```python
from build123d import *


with BuildPart() as f1:
    # F0 (on Top) → F1 (revolve)
    with BuildSketch(Plane.XY):
        Polygon((0, 76.635234), (0, -54.980509), (15.186432, -54.980509), (15.186432, -38.387928), (55.121128, -38.387928), (33.747628, -14.202126), (57.652198, -14.202126), (33.747628, 13.077206), (55.121128, 13.077206), (33.747628, 36.419317), (51.183905, 36.419317), align=None)
    revolve(axis=Axis((0, 10.827363, 0), (0, -1, 0)))


solid = f1.part
```
Geometry check sheet. Reference: the model listing, model coordinates, mm. A direction names the side the tool comes from. Round coordinates to 2 decimals unless told otherwise and drop trailing zeros. Loops run counter-clockwise (first coordinate to the right, second up) from the corner with the lowest first, then second, coordinate; pieces in that order, holes last. Notation, with made-up numbers: (-34, -26) - (25, -26) arc R32 cw to (25, 7) - close; hole circle Ø11 at (11.25, 77). An arc over 180 degrees is marked (long way). Write item = value, one per line. Start each with the question number.
1. Section check B-B on z = 35. Give the number of separate pieces and of enclosed holes in the cut face, then the cut area to 3 significant figures.
2. Section check C-C on y = -44. Enter the section's corners in (x, z), then the cut area to 3 significant figures.
3. Mould release check, pull along Y, two halves, no side actions. Record for faces 4 (the face through (7.8, 70.2, 2.5)), 5 (the face through (-7.541, 35.286, -33.958)), 6 (the face through (-12.05, -46.57, -9.24)): released by +Y, released by -Y, zero draft, split by the parting line, or undercut.
4. Section check A-A on y = 17.5. Enter the section's corners in (x, z).
5. Depth check by flat-ended pin: pin 1 (1.5 mm diameter, centred on x = 29, z = -44, fed in from -Y); pin 2 (8 mm diameter, centred on y = 57, z = -24.5, fed in from -X); pin 3 (5 mm diameter, centred on x = -7.5, z = -10.5, fed in from +Y). Enter the tip coordinate at first touch or a pass-through.
6. Set-up check for faces 1 (the face through (0, -54.981, 0)), 2 (the face through (-11, 36.419, -33)), 3 (the face through (-11, -38.388, -11)): record each of +Z, -Z, +X, -X, +Y, -Y from which the full face is reachable in a straight line by a thin tool's end or side.
7. Thickness scan on line 1 (Y direction, x = -23.5, z = 27); line 2 (Y direction, x = -34, z = -39); line 3 (Y direction, x = -36.5, z = -22). Record the ranges inside material, lowest first.
Working result:
q1.separate_pieces = 4
q1.enclosed_holes = 0
q1.area = 4,530 mm^2
q2.outline = circle Ø30.37 at (0, 0)
q2.area = 725 mm^2
q3.face_4 = released by +Y
q3.face_5 = undercut
q3.face_6 = zero draft
q4.outline = circle Ø102.14 at (0, 0)
q5.pin_1 = -38.39
q5.pin_2 = -18.92
q5.pin_3 = 68.46
q6.face_1 = +Z, -Z, +X, -X, -Y
q6.face_2 = none
q6.face_3 = -Y
q7.line_1 = -38.39 to -16.52, -14.2 to 10.74, 13.08 to 34.18, 36.42 to 48.51
q7.line_2 = -38.39 to -34.56, -14.2 to -7.45, 13.08 to 16.77
q7.line_3 = -38.39 to -24.24, -14.2 to 2.96, 13.08 to 26.73, 36.42 to 43.15
